from build123d import *

# Parameters (mm, degrees)
F0_R     = 44.222485
F0_R_2   = 28.624765
F1_DEPTH = 12.7
F2_R     = 76.2
F2_R_2   = 25.4
F3_DEPTH = 12.7
F4_R     = 76.2
F4_R_2   = 25.4
F5_DEPTH = 12.7


with BuildPart() as f1:
    # F0 (on Front) → F1 (new body, symmetric)
    with BuildSketch(Plane.XZ):
        with BuildLine():
            ThreePointArc((52.951212, -6.35), (53.235671, -3.180662), (53.330604, 0))
            ThreePointArc((53.330604, 0), (53.235671, 3.180662), (52.951212, 6.35))
            ThreePointArc((52.951212, 6.35), (51.513408, 13.802976), (49.032095, 20.976345))
            ThreePointArc((49.032095, 20.976345), (46.185658, 26.665302), (42.682095, 31.974867))
            ThreePointArc((42.682095, 31.974867), (37.710432, 37.710432), (31.974867, 42.682095))
            ThreePointArc((31.974867, 42.682095), (26.665302, 46.185658), (20.976345, 49.032094))
            ThreePointArc((20.976345, 49.032094), (13.802976, 51.513408), (6.35, 52.951212))
            ThreePointArc((6.35, 52.951212), (0, 53.330604), (-6.35, 52.951212))
            ThreePointArc((-6.35, 52.951212), (-13.802976, 51.513408), (-20.976345, 49.032095))
            ThreePointArc((-20.976345, 49.032095), (-26.665302, 46.185658), (-31.974867, 42.682095))
            ThreePointArc((-31.974867, 42.682095), (-37.710432, 37.710432), (-42.682095, 31.974867))
            ThreePointArc((-42.682095, 31.974867), (-46.185658, 26.665302), (-49.032094, 20.976345))
            ThreePointArc((-49.032094, 20.976345), (-51.513408, 13.802976), (-52.951212, 6.35))
            ThreePointArc((-52.951212, 6.35), (-53.330604, 0), (-52.951212, -6.35))
            ThreePointArc((-52.951212, -6.35), (-51.513408, -13.802976), (-49.032095, -20.976345))
            ThreePointArc((-49.032095, -20.976345), (-46.185658, -26.665302), (-42.682095, -31.974867))
            ThreePointArc((-42.682095, -31.974867), (-37.710432, -37.710432), (-31.974867, -42.682095))
            ThreePointArc((-31.974867, -42.682095), (-26.665302, -46.185658), (-20.976345, -49.032094))
            ThreePointArc((-20.976345, -49.032094), (-13.802976, -51.513408), (-6.35, -52.951212))
            ThreePointArc((-6.35, -52.951212), (0, -53.330604), (6.35, -52.951212))
            ThreePointArc((6.35, -52.951212), (13.802976, -51.513408), (20.976345, -49.032095))
            ThreePointArc((20.976345, -49.032095), (26.665302, -46.185658), (31.974867, -42.682095))
            ThreePointArc((31.974867, -42.682095), (37.710432, -37.710432), (42.682095, -31.974867))
            ThreePointArc((42.682095, -31.974867), (46.185658, -26.665302), (49.032094, -20.976345))
            ThreePointArc((49.032094, -20.976345), (51.513408, -13.802976), (52.951212, -6.35))
        make_face()
        Circle(F0_R, mode=Mode.SUBTRACT)
        with BuildLine():
            Line((72.380604, 0), (53.330604, 0))
            ThreePointArc((53.330604, 0), (53.235671, -3.180662), (52.951212, -6.35))
            Line((52.951212, -6.35), (57.618118, -6.35))
            ThreePointArc((57.618118, -6.35), (58.493309, -6.255681), (59.364783, -6.131635))
            ThreePointArc((59.364783, -6.131635), (66.307622, -3.989055), (72.380604, 0))
        make_face()
        with BuildLine():
            ThreePointArc((52.951212, 6.35), (53.235671, 3.180662), (53.330604, 0))
            Line((53.330604, 0), (72.380604, 0))
            ThreePointArc((72.380604, 0), (66.608564, 4.174833), (59.825179, 6.35))
            Line((59.825179, 6.35), (59.341823, 6.35))
            ThreePointArc((59.341823, 6.35), (59.338073, 6.384943), (59.334303, 6.419883))
            ThreePointArc((59.334303, 6.419883), (56.140283, 6.610983), (52.951212, 6.35))
        make_face()
        with BuildLine():
            Line((57.618118, -6.35), (52.951212, -6.35))
            ThreePointArc((52.951212, -6.35), (55.284665, -6.455472), (57.618118, -6.35))
        make_face()
        with BuildLine():
            ThreePointArc((42.682095, 31.974867), (46.185658, 26.665302), (49.032095, 20.976345))
            ThreePointArc((49.032095, 20.976345), (57.424424, 27.177577), (62.683442, 36.190302))
            ThreePointArc((62.683442, 36.190302), (52.180088, 36.467695), (42.682095, 31.974867))
        make_face()
        with BuildLine():
            ThreePointArc((59.825179, 6.35), (59.579932, 6.386285), (59.334303, 6.419883))
            ThreePointArc((59.334303, 6.419883), (59.338073, 6.384943), (59.341823, 6.35))
            Line((59.341823, 6.35), (59.825179, 6.35))
        make_face()
        with BuildLine():
            ThreePointArc((62.683442, -36.190302), (57.671995, -26.955434), (49.032094, -20.976345))
            ThreePointArc((49.032094, -20.976345), (46.185658, -26.665302), (42.682095, -31.974867))
            ThreePointArc((42.682095, -31.974867), (52.248684, -36.142222), (62.683442, -36.190302))
        make_face()
        with BuildLine():
            ThreePointArc((59.364783, -6.131635), (58.493309, -6.255681), (57.618118, -6.35))
            Line((57.618118, -6.35), (59.341823, -6.35))
            ThreePointArc((59.341823, -6.35), (59.353403, -6.240828), (59.364783, -6.131635))
        make_face()
        with BuildLine():
            ThreePointArc((20.976345, 49.032094), (26.665302, 46.185658), (31.974867, 42.682095))
            ThreePointArc((31.974867, 42.682095), (36.142222, 52.248684), (36.190302, 62.683442))
            ThreePointArc((36.190302, 62.683442), (26.955434, 57.671995), (20.976345, 49.032094))
        make_face()
        with BuildLine():
            ThreePointArc((36.190302, -62.683442), (36.467695, -52.180088), (31.974867, -42.682095))
            ThreePointArc((31.974867, -42.682095), (26.665302, -46.185658), (20.976345, -49.032095))
            ThreePointArc((20.976345, -49.032095), (27.177577, -57.424424), (36.190302, -62.683442))
        make_face()
        with BuildLine():
            ThreePointArc((-6.35, 52.951212), (0, 53.330604), (6.35, 52.951212))
            ThreePointArc((6.35, 52.951212), (5.17574, 63.319798), (0, 72.380604))
            ThreePointArc((0, 72.380604), (-5.491907, 63.423129), (-6.35, 52.951212))
        make_face()
        with BuildLine():
            ThreePointArc((0, -72.380604), (5.491907, -63.423129), (6.35, -52.951212))
            ThreePointArc((6.35, -52.951212), (0, -53.330604), (-6.35, -52.951212))
            ThreePointArc((-6.35, -52.951212), (-5.17574, -63.319798), (0, -72.380604))
        make_face()
        with BuildLine():
            ThreePointArc((-31.974867, 42.682095), (-26.665302, 46.185658), (-20.976345, 49.032095))
            ThreePointArc((-20.976345, 49.032095), (-27.177577, 57.424424), (-36.190302, 62.683442))
            ThreePointArc((-36.190302, 62.683442), (-36.467695, 52.180088), (-31.974867, 42.682095))
        make_face()
        with BuildLine():
            ThreePointArc((-36.190302, -62.683442), (-26.955434, -57.671995), (-20.976345, -49.032094))
            ThreePointArc((-20.976345, -49.032094), (-26.665302, -46.185658), (-31.974867, -42.682095))
            ThreePointArc((-31.974867, -42.682095), (-36.142222, -52.248684), (-36.190302, -62.683442))
        make_face()
        with BuildLine():
            ThreePointArc((-49.032094, 20.976345), (-46.185658, 26.665302), (-42.682095, 31.974867))
            ThreePointArc((-42.682095, 31.974867), (-52.248684, 36.142222), (-62.683442, 36.190302))
            ThreePointArc((-62.683442, 36.190302), (-57.671995, 26.955434), (-49.032094, 20.976345))
        make_face()
        with BuildLine():
            ThreePointArc((-62.683442, -36.190302), (-52.180088, -36.467695), (-42.682095, -31.974867))
            ThreePointArc((-42.682095, -31.974867), (-46.185658, -26.665302), (-49.032095, -20.976345))
            ThreePointArc((-49.032095, -20.976345), (-57.424424, -27.177577), (-62.683442, -36.190302))
        make_face()
        with BuildLine():
            ThreePointArc((-52.951212, -6.35), (-53.330604, 0), (-52.951212, 6.35))
            ThreePointArc((-52.951212, 6.35), (-63.319798, 5.17574), (-72.380604, 0))
            ThreePointArc((-72.380604, 0), (-63.423129, -5.491907), (-52.951212, -6.35))
        make_face()
        Circle(F0_R)
        Circle(F0_R_2, mode=Mode.SUBTRACT)
    extrude(amount=F1_DEPTH, both=True)

    # F2 (on face) → F3 (join)
    with BuildSketch(Plane.XZ.offset(12.7)):
        Circle(F2_R)
        Circle(F2_R_2, mode=Mode.SUBTRACT)
    extrude(amount=F3_DEPTH)

    # F4 (on face) → F5 (join)
    with BuildSketch(Plane(origin=(0, 12.7, 0), x_dir=(-1, 0, 0), z_dir=(0, 1, 0))):
        Circle(F4_R)
        Circle(F4_R_2, mode=Mode.SUBTRACT)
    extrude(amount=F5_DEPTH)


solid = f1.part
Can you work these out from the model? Positions are in its coordinate system, mm. A direction names the side the tool comes from. Round coordinates to 2 decimals unless told otherwise and drop trailing zeros. Order: outer loops, then holes, each group sorted by start corner. A loop starts at its lowest first (then second) coordinate and runs counter-clockwise, first axis right, second up. Notation, with made-up numbers: (60.5, 52) - (78.5, 52) arc R11 ccw to (78.5, 61) - close; hole circle Ø7 at (46.25, 54). An arc over 180 degrees is marked (long way). Answer in a Markdown table with one row per item.
(1) Suppose I cut it at A-A, the plane x = -4. Please give me the cut outline in (y, z), plus the area to 3 significant figures.
From the geometry:
| item | result |
|---|---|
| outline | (-25.4, -76.09) - (-12.7, -76.09) - (-12.7, -66.28) - (12.7, -66.28) - (12.7, -76.09) - (25.4, -76.09) - (25.4, -25.08) - (12.7, -25.08) - (12.7, -28.34) - (-12.7, -28.34) - (-12.7, -25.08) - (-25.4, -25.08) - close; (-25.4, 25.08) - (-12.7, 25.08) - (-12.7, 28.34) - (12.7, 28.34) - (12.7, 25.08) - (25.4, 25.08) - (25.4, 76.09) - (12.7, 76.09) - (12.7, 66.95) - (-12.7, 66.95) - (-12.7, 76.09) - (-25.4, 76.09) - close |
| area | 4,540 mm2 |
(2) Suppose I cut it at B-B, the plane z = 57.5. Please give me the cut outline in (x, y).
From the geometry:
| item | result |
|---|---|
| outline | (-50, -25.4) - (50, -25.4) - (50, -12.7) - (36.7, -12.7) - (36.7, 12.7) - (50, 12.7) - (50, 25.4) - (-50, 25.4) - (-50, 12.7) - (-36.95, 12.7) - (-36.95, -12.7) - (-50, -12.7) - close; hole (-27.26, -12.7) - (-6.59, -12.7) - (-6.59, 12.7) - (-27.26, 12.7) - close; hole (6.36, -12.7) - (26.77, -12.7) - (26.77, 12.7) - (6.36, 12.7) - close |
(3) Please list where these lines run through material, in increasing order: L1, parallel to Z at x = 0, y = 21.75; L2, parallel to Y at x = -25.5, z = -9.5; L3, parallel to Z at x = 59, y = 10. Write a range as from..to.
From the geometry:
| item | result |
|---|---|
| L1 | z = -76.2..-25.4, 25.4..76.2 |
| L2 | y = -25.4..-12.7, 12.7..25.4 |
| L3 | z = -36.66..-28.58, -6.35..6.46, 29.11..36.85 |
(4) Which directions (+Z, -Z, +X, -X, +Y, -Y) give clear straight access to the entire face, cutting with the end or side of a thin tool? Please do faces 3 (the face through (-57.33, -0.18, -27.07)), 4 (the face through (-52.33, -0.18, -36.5)), 5 (the face through (-17, -12.7, 51)), 6 (the face through (27.1, -0.2, 57.8)).
From the geometry:
| item | result |
|---|---|
| face 3 | -X |
| face 4 | -Z |
| face 5 | none |
| face 6 | +Z |
(5) For P1, Ø12, axis at y = 4, z = -13.5, coming from the -X side; P2, Ø1.4, axis at x = 59, y = -4.5, coming from the -Z side; P3, Ø1, axis at x = -40.5, y = 20, coming from the +Z side, each with a flat end and sliding along its axis, tell me the tip position at first contact or that it passes through.
From the geometry:
| item | result |
|---|---|
| P1 | stops at x = -52.8 |
| P2 | stops at z = -36.69 |
| P3 | stops at z = 64.86 |
(6) If we mould it in two halves opening along Y, with no side actions, what happens to faces 1 (the face through (-63.564, -0.178, -5.445)), 2 (the face through (5.506, 18.961, -24.796))? For each: released by +Y, released by -Y, zero draft, split by the parting line, or undercut.
From the geometry:
| item | result |
|---|---|
| face 1 | undercut |
| face 2 | zero draft |
(7) Suppose I cut it at C-C, the plane x = 15. Please give me the cut outline in (y, z), plus the area to 3 significant figures.
From the geometry:
| item | result |
|---|---|
| outline | (-25.4, -74.71) - (-12.7, -74.71) - (-12.7, -51.18) - (12.7, -51.18) - (12.7, -74.71) - (25.4, -74.71) - (25.4, -20.5) - (12.7, -20.5) - (12.7, -24.38) - (-12.7, -24.38) - (-12.7, -20.5) - (-25.4, -20.5) - close; (-25.4, 20.5) - (-12.7, 20.5) - (-12.7, 24.38) - (12.7, 24.38) - (12.7, 20.5) - (25.4, 20.5) - (25.4, 74.71) - (12.7, 74.71) - (12.7, 51.18) - (-12.7, 51.18) - (-12.7, 74.71) - (-25.4, 74.71) - close |
| area | 4,120 mm2 |
(8) Suppose I cut it at D-D, the plane z = -59. Please give me the cut outline in (x, y), plus the area to 3 significant figures.
From the geometry:
| item | result |
|---|---|
| outline | (-48.22, -25.4) - (48.22, -25.4) - (48.22, -12.7) - (36.85, -12.7) - (36.85, 12.7) - (48.22, 12.7) - (48.22, 25.4) - (-48.22, 25.4) - (-48.22, 12.7) - (-36.66, 12.7) - (-36.66, -12.7) - (-48.22, -12.7) - close; hole (-28.58, -12.7) - (-6.19, -12.7) - (-6.19, 12.7) - (-28.58, 12.7) - close; hole (6.46, -12.7) - (29.11, -12.7) - (29.11, 12.7) - (6.46, 12.7) - close |
| area | 3,170 mm2 |
